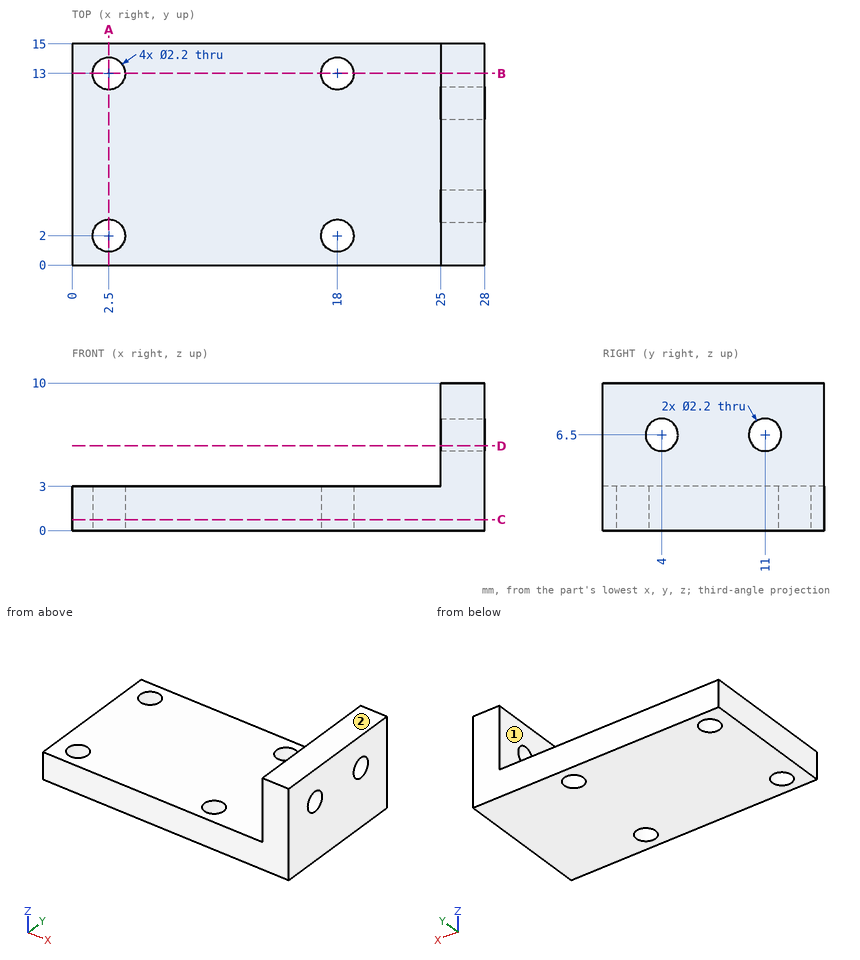
The drawing under review shows one solid part. Ordinate dimensions are in mm from its lowest x, y, z. A direction names the side the tool comes from. Round coordinates to 2 decimals unless told otherwise and drop trailing zeros. Write each loop counter-clockwise with the first axis right and the second up, starting at its lowest first coordinate (ties: lowest second). Pieces come first, ordered by that corner, then holes. Notation, with made-up numbers: (68.5, 5) - (114.5, 5) arc R32 ccw to (114.5, 31) - close; hole circle Ø5 at (-36, -3). An arc over 180 degrees is marked (long way). Use a Markdown table: item, result. Add a question column.
1. We need section D-D (z = 5.75). State the section outline as (x, y) points.
2. We need section B-B (y = 13). State the section outline as (x, z) points, then the cut area to 3 significant figures.
3. We need section C-C (z = 0.75). State the section outline as (x, y) points.
4. We need section A-A (x = 2.5). State the section outline as (y, z) points, then the cut area to 3 significant figures.
5. For the marked faces 1 and 2, list the 3-axis set-ups (+Z, -Z, +X, -X, +Y, -Y) from which the entire face can be reached by the end or side of a thin tool; tool diameter is ignored.
6. Wall thickness on probe 1 along X at (y, z) = (13, 0.9); probe 2 along Y at (x, z) = (18, 2.3); probe 3 along Y at (x, z) = (26.5, 6.5): over which ranges is each line inside the solid? List them lowest first.
7. Clearance check with flat-ended pins moving along their axes: pin 1 (2.5 mm diameter, centred on x = 2.5, y = 13, fed in from -Z); pin 2 (4 mm diameter, centred on x = 3.5, y = 3.5, fed in from +Z); pin 3 (2 mm diameter, centred on y = 7.5, z = 6, fed in from -X). State where each tip first meets the part, or that it passes through.
Output:
| question | item | result |
|---|---|---|
| 1 | outline | (25, 0) - (28, 0) - (28, 3.2) - (25, 3.2) - close; (25, 4.8) - (28, 4.8) - (28, 10.2) - (25, 10.2) - close; (25, 11.8) - (28, 11.8) - (28, 15) - (25, 15) - close |
| 2 | outline | (0, 0) - (1.4, 0) - (1.4, 3) - (0, 3) - close; (3.6, 0) - (16.9, 0) - (16.9, 3) - (3.6, 3) - close; (19.1, 0) - (28, 0) - (28, 10) - (25, 10) - (25, 3) - (19.1, 3) - close |
| 2 | area | 91.8 mm2 |
| 3 | outline | (0, 0) - (28, 0) - (28, 15) - (0, 15) - close; hole circle Ø2.2 at (2.5, 2); hole circle Ø2.2 at (2.5, 13); hole circle Ø2.2 at (18, 2); hole circle Ø2.2 at (18, 13) |
| 4 | outline | (0, 0) - (0.9, 0) - (0.9, 3) - (0, 3) - close; (3.1, 0) - (11.9, 0) - (11.9, 3) - (3.1, 3) - close; (14.1, 0) - (15, 0) - (15, 3) - (14.1, 3) - close |
| 4 | area | 31.8 mm2 |
| 5 | face 1 | +Z, -X, +Y, -Y |
| 5 | face 2 | +Z, +X, -X, +Y, -Y |
| 6 | probe 1 | x = 0 to 1.4, 3.6 to 16.9, 19.1 to 28 |
| 6 | probe 2 | y = 0 to 0.9, 3.1 to 11.9, 14.1 to 15 |
| 6 | probe 3 | y = 0 to 2.9, 5.1 to 9.9, 12.1 to 15 |
| 7 | pin 1 | stops at z = 0 |
| 7 | pin 2 | stops at z = 3 |
| 7 | pin 3 | stops at x = 25 |
